For this review, take the finished solid that the model builds, in its own axes (mm). A direction names the side the tool comes from. Round coordinates to 2 decimals unless told otherwise and drop trailing zeros. Write each loop counter-clockwise with the first axis right and the second up, starting at its lowest first coordinate (ties: lowest second). Pieces come first, ordered by that corner, then holes. Notation, with made-up numbers: M -33,31.5 L 0,31.5 A35 cw 0,63.5 Z; hole C 21.25,10 d2. An arc over 180 degrees is marked long. Answer in a Markdown table with one row per item.
```python
from build123d import *

# Parameters (mm, degrees)
F0_R     = 55
F1_DEPTH = 5
F2_R     = 3
F3_R     = 1.99999
F4_R     = 49.5
F5_DEPTH = 5
F6_R     = 49.5
F6_R_2   = 42.5
F7_DEPTH = 2
F8_R     = 1.99999


# Not quite as in the source:
# - a fillet or chamfer is up to 0.001 mm smaller than in the source, because OpenCascade refuses the exact size


with BuildPart() as f1:
    # F0 (on Top) → F1 (new body)
    with BuildSketch(Plane.XY):
        Circle(F0_R)
    extrude(amount=-F1_DEPTH)

    # F2
    f2_edges = [f1.edges().sort_by_distance(p)[0] for p in [
        (-55, 0, -5),
    ]]
    fillet(f2_edges, radius=F2_R)

    # F3 (radius 2 in the source; OpenCascade refuses exactly that, so slightly less here)
    f3_edges = [f1.edges().sort_by_distance(p)[0] for p in [
        (-55, 0, 0),
    ]]
    fillet(f3_edges, radius=F3_R)

    # F4 (on Top) → F5 (cut)
    with BuildSketch(Plane.XY):
        Circle(F4_R)
    extrude(amount=-F5_DEPTH, mode=Mode.SUBTRACT)

    # F6 (on face) → F7 (join)
    with BuildSketch(Plane(origin=(0, 0, -5), x_dir=(1, 0, 0), z_dir=(0, 0, -1))):
        Circle(F6_R)
        Circle(F6_R_2, mode=Mode.SUBTRACT)
    extrude(amount=-F7_DEPTH)

    # F8 (radius 2 in the source; OpenCascade refuses exactly that, so slightly less here)
    f8_edges = [f1.edges().sort_by_distance(p)[0] for p in [
        (-42.5, 0, -3),
    ]]
    fillet(f8_edges, radius=F8_R)


solid = f1.part
```
Q1. For probe 1 along Y at (x, z) = (0, -1.85); probe 2 along Y at (x, z) = (0, -0.85); probe 3 along X at (y, z) = (29, -4.3), list the stretches that pass through material, from the lowest coordinate up.
Found:
| item | result |
|---|---|
| probe 1 | -54.99 to -49.5, 49.5 to 54.99 |
| probe 2 | -54.64 to -49.5, 49.5 to 54.64 |
| probe 3 | -45.46 to -31.24, 31.24 to 45.46 |
Q2. Take a section at C-C (z = -1). State the section outline as (x, y) points, then the cut area to 3 significant figures.
Found:
| item | result |
|---|---|
| outline | C 0,0 d109.46; hole C 0,0 d99 |
| area | 1,710 mm² |
Q3. Mouldability with a two-part tool opening along X and no side actions: class faces 1 (the face through (-43, 0, -5)), 2 (the face through (-6.44, 49.08, -1.48)) as +X half, -X half, draft (parallel to the pull), parting line (faces both ways), or undercut.
Found:
| item | result |
|---|---|
| face 1 | draft |
| face 2 | undercut |
Q4. Insertion check: P1, Ø1, axis at x = 34.5, y = 27.5, coming from the +Z side; P2, Ø2, axis at x = 40.5, y = -13.5, coming from the +Z side. Each pin has a flat end and moves straight along its axis. Give the tip position at first contact, or say it passes through.
Found:
| item | result |
|---|---|
| P1 | z = -3 |
| P2 | z = -3.17 |
Q5. Machinability: for faces 3 (the face through (-47.4, -15.5, 0)), 4 (the face through (-41, -19, -3)), which of the approach directions +Z, -Z, +X, -X, +Y, -Y give a long, thin tool a straight path to every point of the face, cutting with its end or side? Answer none if there is none.
Found:
| item | result |
|---|---|
| face 3 | +Z, +X, -X, +Y, -Y |
| face 4 | +Z |
